Check sheet for the modelled part. Datum: model origin and axes. Units: mm. A direction names the side the tool comes from. Give positions to 0.01 mm unless a question says otherwise; leave off trailing zeros. Write each loop counter-clockwise with the first axis right and the second up, starting at its lowest first coordinate (ties: lowest second). Pieces come first, ordered by that corner, then holes. Notation, with made-up numbers: (77.25, -15.75) -> (135.25, -15.75) arc R36 cw to (135.25, 22.25) -> close; hole circle Ø11 at (-14.75, 47). An arc over 180 degrees is marked (long way). Use a Markdown table: item, result. Add a question column.
1. Scan lines: probe 1 along X at (y, z) = (112, 23); probe 2 along Y at (x, z) = (56, 12); probe 3 along X at (y, z) = (-130, 22). Record each from-to range of solid material in increasing order. Write a range as [from, to].
2. Cross-section at C-C (y = 15). Enter the section's corners in (x, z).
3. Release check for a two-part mould opening along Y. For faces 4 (the flat face through (212, -79.883, 12)), 5 (the flat face through (-81.779, -147, 12)), 6 (the flat face through (98.221, 83, 13)) record: released by +Y, released by -Y, zero draft, split by the parting line, or undercut.
4. Cross-section at B-B (z = 19.5). Enter the section's corners in (x, y).
5. Set-up check for faces 1 (the flat face through (198.221, 177, 12)), 2 (the flat face through (18.221, 83, 13)), 3 (the flat face through (198.221, -147, 12)): record each of +Z, -Z, +X, -X, +Y, -Y from which the full face is reachable in a straight line by a thin tool's end or side.
6. Cross-section at A-A (y = 131). Enter the section's corners in (x, z).
7. Gauge pin test, flat ends, axial feed: P1, Ø7.5, axis at y = -131, z = 13.5, coming from the -X side; P2, Ø12.5, axis at x = -94.5, z = 16.5, coming from the -Y side; P3, Ø3, axis at y = 124, z = 17, coming from the +X side. Record the tip position at first contact, or that the pin passes through.
from build123d import *

# Parameters (mm, degrees)
SKETCH1_W           = 336
SKETCH1_H           = 456
BOSS_EXTRUDE1_DEPTH = 25
SKETCH3_W           = 28
SKETCH3_H           = 132
CUT_EXTRUDE1_DEPTH  = 25
SKETCH4_W           = 80
SKETCH4_H           = 160
CUT_EXTRUDE2_DEPTH  = 25


with BuildPart() as part:
    # Sketch1 → Boss-Extrude1 (new body)
    with BuildSketch(Plane.XY):
        with Locations((58.220689655, 16.117241379)):
            Rectangle(SKETCH1_W, SKETCH1_H)
    extrude(amount=BOSS_EXTRUDE1_DEPTH)

    # Sketch3 → Cut-Extrude1 (cut)
    with BuildSketch(Plane.XY):
        with Locations((-95.779310345, 178.117241379)):
            Rectangle(SKETCH3_W, SKETCH3_H)
        with Locations((212.220689655, 178.117241379)):
            Rectangle(SKETCH3_W, SKETCH3_H)
        with Locations((212.220689655, -145.882758621)):
            Rectangle(SKETCH3_W, SKETCH3_H)
        with Locations((-95.779310345, -145.882758621)):
            Rectangle(SKETCH3_W, SKETCH3_H)
    extrude(amount=CUT_EXTRUDE1_DEPTH, mode=Mode.SUBTRACT)

    # Sketch4 → Cut-Extrude2 (cut)
    with BuildSketch(Plane.XY.offset(25)):
        with Locations((58.220689655, 84.117241379)):
            Rectangle(SKETCH4_W, SKETCH4_H)
    extrude(amount=-CUT_EXTRUDE2_DEPTH, mode=Mode.SUBTRACT)


solid = part.part
Worked answers:
| question | item | result |
|---|---|---|
| 1 | probe 1 | x = [-109.78, 18.22], [98.22, 226.22] |
| 1 | probe 2 | y = [-211.88, 4.12], [164.12, 244.12] |
| 1 | probe 3 | x = [-81.78, 198.22] |
| 2 | outline | (-109.78, 0) -> (18.22, 0) -> (18.22, 25) -> (-109.78, 25) -> close; (98.22, 0) -> (226.22, 0) -> (226.22, 25) -> (98.22, 25) -> close |
| 3 | face 4 | released by -Y |
| 3 | face 5 | zero draft |
| 3 | face 6 | undercut |
| 4 | outline | (-109.78, -79.88) -> (-81.78, -79.88) -> (-81.78, -211.88) -> (198.22, -211.88) -> (198.22, -79.88) -> (226.22, -79.88) -> (226.22, 112.12) -> (198.22, 112.12) -> (198.22, 244.12) -> (-81.78, 244.12) -> (-81.78, 112.12) -> (-109.78, 112.12) -> close; hole (18.22, 4.12) -> (98.22, 4.12) -> (98.22, 164.12) -> (18.22, 164.12) -> close |
| 5 | face 1 | +Z, -Z, +X, +Y |
| 5 | face 2 | +Z, -Z |
| 5 | face 3 | +Z, -Z, +X, -Y |
| 6 | outline | (-81.78, 0) -> (18.22, 0) -> (18.22, 25) -> (-81.78, 25) -> close; (98.22, 0) -> (198.22, 0) -> (198.22, 25) -> (98.22, 25) -> close |
| 7 | P1 | stops at x = -81.78 |
| 7 | P2 | stops at y = -79.88 |
| 7 | P3 | stops at x = 198.22 |
